from build123d import *

# Parameters (mm, degrees)
SKETCH1_R                                           = 30
BOSS_EXTRUDE1_DEPTH                                 = 15
SKETCH10_R                                          = 5
CUT_EXTRUDE2_DEPTH                                  = 15
CBORE_FOR_M4_HEX_SOCKET_HEAD_CAP_SCREW3_D           = 4.5
CBORE_FOR_M4_HEX_SOCKET_HEAD_CAP_SCREW3_DEPTH       = 15
CBORE_FOR_M4_HEX_SOCKET_HEAD_CAP_SCREW3_CBORE_D     = 8
CBORE_FOR_M4_HEX_SOCKET_HEAD_CAP_SCREW3_CBORE_DEPTH = 4.4


with BuildPart() as part:
    # Sketch1 → Boss-Extrude1 (new body)
    with BuildSketch(Plane(origin=(0, 0, 0), x_dir=(1, 0, 0), z_dir=(0, 1, 0))):
        with Locations((121.722144349, 83.935831041)):
            Circle(SKETCH1_R)
    extrude(amount=BOSS_EXTRUDE1_DEPTH)

    # Sketch10 → Cut-Extrude2 (cut)
    with BuildSketch(Plane(origin=(0, 15, 0), x_dir=(1, 0, 0), z_dir=(0, 1, 0))):
        with Locations((121.722144349, 83.935831041)):
            Circle(SKETCH10_R)
    extrude(amount=-CUT_EXTRUDE2_DEPTH, mode=Mode.SUBTRACT)

    # CBORE for M4 Hex Socket Head Cap Screw3
    with Locations(Plane(origin=(132.222144349, 15, -102.935831041), x_dir=(0, 0, 1), z_dir=(0, 1, 0))):
        with Locations((0, 0), (0, -21)):
            CounterBoreHole(CBORE_FOR_M4_HEX_SOCKET_HEAD_CAP_SCREW3_D / 2, CBORE_FOR_M4_HEX_SOCKET_HEAD_CAP_SCREW3_CBORE_D / 2, CBORE_FOR_M4_HEX_SOCKET_HEAD_CAP_SCREW3_CBORE_DEPTH, depth=CBORE_FOR_M4_HEX_SOCKET_HEAD_CAP_SCREW3_DEPTH)


solid = part.part
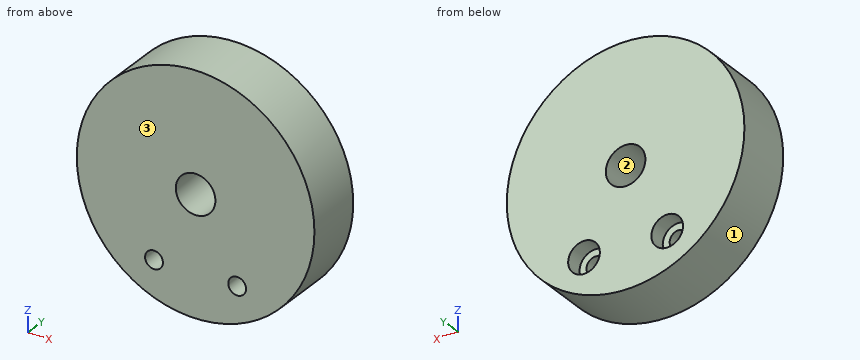
Design review of the part built by this model. Coordinates are the model's own, in mm. Face numbers are marked on the shaded views. Coordinates: 2 decimals unless noted, no trailing zeros. Order: outer loops, then holes, each group sorted by start corner. A loop starts at its lowest first (then second) coordinate and runs counter-clockwise, first axis right, second up.
Item 1: Take a section at A-A, the plane x = 124.5. Write out the cut boundary in (y, z), then the cut area to 3 significant figures.
Item 2: Take a section at B-B, the plane x = 135.5. Write out the cut boundary in (y, z).
Item 3: Take a section at C-C, the plane z = -59.5. Write out the cut boundary in (x, y).
Item 4: The part is to be moulded in two halves that separate along X. For the marked faces 1, 2 and 3, say which applies: pulls with the +X half, pulls with the -X half, needs draft (parallel to the pull), parting line crosses it, or undercut.
Item 5: Take a section at D-D, the plane y = 3.5. Write out the cut boundary in (x, z), then the cut area to 3 significant figures.
Item 6: For pin 1 Ø3.5 at (x, z) = (111.22, -102.94) entering from +Y; pin 2 Ø1 at (x, y) = (104.5, 12) entering from -Z; pin 3 Ø6 at (y, z) = (6, -103) entering from -X; pin 4 Ø8 at (y, z) = (2, -97) entering from -X, all flat-tipped, find the tip position at first contact; note any pin that passes through.
Item 7: For line 1 (Z direction, x = 124, y = 14.25); line 2 (X direction, y = 13, z = -104.5); line 3 (X direction, y = 14.25, z = -85), list the stretches that pass through material, from the lowest coordinate up.
The answers:
1. outline: (0, -113.81) - (15, -113.81) - (15, -88.09) - (0, -88.09) - close; (0, -79.78) - (15, -79.78) - (15, -54.06) - (0, -54.06) - close
1. area: 771 mm2
2. outline: (0, -110.58) - (15, -110.58) - (15, -105.23) - (10.6, -105.23) - (10.6, -100.64) - (15, -100.64) - (15, -57.29) - (0, -57.29) - close
3. outline: (104.32, 0) - (139.13, 0) - (139.13, 15) - (104.32, 15) - close
4. face 1: parting line crosses it
4. face 2: undercut
4. face 3: needs draft
5. outline: circle Ø60 at (121.72, -83.94); hole circle Ø4.5 at (111.22, -102.94); hole circle Ø10 at (121.72, -83.94); hole circle Ø4.5 at (132.22, -102.94)
5. area: 2,720 mm2
6. pin 1: passes through
6. pin 2: stops at z = -108.84
6. pin 3: stops at x = 96.39
6. pin 4: stops at x = 93.12
7. line 1: z = -113.85 to -88.39, -79.48 to -54.02
7. line 2: x = 99.88 to 107.54, 114.9 to 128.54, 135.9 to 143.57
7. line 3: x = 91.74 to 116.84, 126.61 to 151.7
